```python
from build123d import *

# Parameters (mm, degrees)
SKETCH2_W               = 12.7
SKETCH2_H               = 6.35
BOSS_EXTRUDE1_DEPTH     = 9.525
EXTRUDE_THIN1_DEPTH     = 9.525
SKETCH4_R               = 4.370013209
CUT_EXTRUDE1_DEPTH      = 9.292796384
CUT_EXTRUDE1_DEPTH_BACK = 9.129454628
EXTRUDE_THIN3_DEPTH     = 1.27


with BuildPart() as part:
    # Sketch2 → Boss-Extrude1 (new body)
    with BuildSketch(Plane(origin=(0, 0, 0), x_dir=(1, 0, 0), z_dir=(0, 1, 0))):
        with Locations((0, -3.175)):
            Rectangle(SKETCH2_W, SKETCH2_H)
    extrude(amount=-BOSS_EXTRUDE1_DEPTH)

    # Sketch3 → Extrude-Thin1 (add)
    with BuildSketch(Plane(origin=(0, 0, 0), x_dir=(1, 0, 0), z_dir=(0, 1, 0))):
        with BuildLine():
            ThreePointArc((-6.979657819, -9.309768687), (0.081670878, -7.62), (7.142999576, -9.309768687))
            Line((7.142999576, -9.309768687), (8.292796384, -7.044913879))
            ThreePointArc((8.292796384, -7.044913879), (0.081670878, -5.08), (-8.129454628, -7.044913879))
            Line((-8.129454628, -7.044913879), (-6.979657819, -9.309768687))
        make_face()
    extrude(amount=-EXTRUDE_THIN1_DEPTH)

    # Sketch4 → Cut-Extrude1 (cut, two sides)
    with BuildSketch(Plane(origin=(0, 0, 0), x_dir=(0, 0, -1), z_dir=(1, 0, 0))) as cut_extrude1_sk:
        with Locations((-1.517033844, -4.7625)):
            Circle(SKETCH4_R)
    extrude(amount=CUT_EXTRUDE1_DEPTH, mode=Mode.SUBTRACT)
    extrude(cut_extrude1_sk.sketch, amount=-CUT_EXTRUDE1_DEPTH_BACK, mode=Mode.SUBTRACT)

    # Sketch6 → Extrude-Thin3 (add)
    with BuildSketch(Plane.XY):
        with BuildLine():
            ThreePointArc((-6.433087898, 0), (-0.041543949, 6.391543949), (6.35, 0))
            Line((6.35, 0), (5.08, 0))
            ThreePointArc((5.08, 0), (-0.041543949, 5.121543949), (-5.163087898, 0))
            Line((-5.163087898, 0), (-6.433087898, 0))
        make_face()
    extrude(amount=EXTRUDE_THIN3_DEPTH)


solid = part.part
```
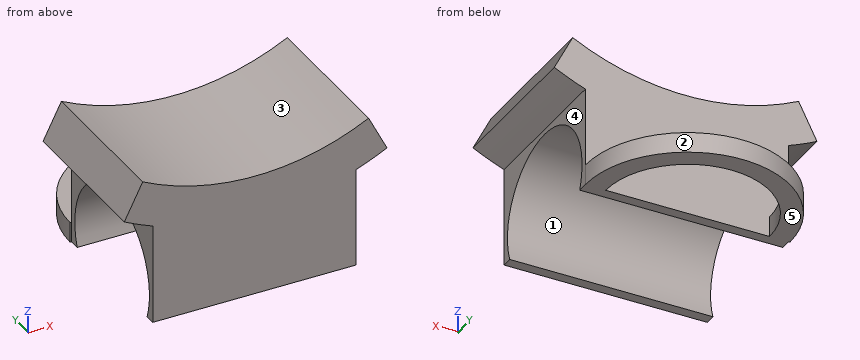
Verification items for the finished model (mm, model axes). Face numbers are marked on the shaded views. A direction names the side the tool comes from. Round coordinates to 2 decimals unless told otherwise and drop trailing zeros. Write each loop counter-clockwise with the first axis right and the second up, starting at its lowest first coordinate (ties: lowest second). Pieces come first, ordered by that corner, then holes. Notation, with made-up numbers: (67.5, -10) -> (125.5, -10) arc R20 cw to (125.5, 26) -> close; hole circle Ø2 at (57, -0.5). An arc over 180 degrees is marked (long way). Write each question's results on one line, items separated by ' | '. Start each with the question number.
1. Material ranges on probe 1 along Y at (x, z) = (-5, 1.5) (3 decimals); probe 2 along Z at (x, y) = (2.5, 5.5); probe 3 along X at (y, z) = (-7.75, 4.75), recorded low to high. Write a range as from..to.
2. Cross-section at B-B (y = 2.25). Enter the section's corners in (x, z), then the cut area to 3 significant figures.
3. Depth check by flat-ended pin: P1, Ø3, axis at x = -4, z = 5, coming from the +Y side; P2, Ø1.9, axis at y = -7, z = 2, coming from the +X side; P3, Ø5, axis at x = 4.5, y = -2.5, coming from the +Z side; P4, Ø2, axis at x = -1, y = -4, coming from the -Z side. Enter the tip coordinate at first touch or a pass-through.
4. Draft check along Z on the marked faces 1, 2 and 3. Enter one of: +Z half, -Z half, draft (parallel to the pull), parting line (faces both ways), or undercut.
5. Cross-section at C-C (z = 4.25). Enter the section's corners in (x, y) (3 decimals), then the cut area to 3 significant figures.
6. Cross-section at A-A (x = 2.5). Enter the section's corners in (y, z) (1 decimal).
7. Set-up check for the marked faces 4 and 5: record each of +Z, -Z, +X, -X, +Y, -Y from which the full face is reachable in a straight line by a thin tool's end or side.
8. Cross-section at D-D (y = -3.75). Enter the section's corners in (x, z).
Solutions:
1) probe 1: y = -9.525..-9.132, -0.393..0 | probe 2: z = 0..1.27 | probe 3: x = -6.35..6.35
2) outline: (-6.02, 0) -> (-4.64, 0) -> (-4.64, 1.27) -> (-6.02, 1.27) -> close; (4.56, 0) -> (5.94, 0) -> (5.94, 1.27) -> (4.56, 1.27) -> close | area: 3.51 mm2
3) P1: stops at y = 0 | P2: passes through | P3: stops at z = 9.24 | P4: stops at z = 5.52
4) face 1: undercut | face 2: draft | face 3: +Z half
5) outline: (-6.35, -9.525) -> (6.35, -9.525) -> (6.35, -8.172) -> (-6.35, -8.172) -> close; (-6.35, -1.353) -> (6.35, -1.353) -> (6.35, 0) -> (-6.35, 0) -> close | area: 34.4 mm2
6) outline: (-9.5, 0) -> (-8.9, 0) arc R4.4 cw (long way) to (-0.7, 0) -> (0, 0) -> (0, 7.8) -> (-9.5, 7.8) -> close; (4.4, 0) -> (5.9, 0) -> (5.9, 1.3) -> (4.4, 1.3) -> close
7) face 4: -Z, +X, +Y, -Y | face 5: -Z, +X, -X, +Y, -Y
8) outline: (-8.13, 7.04) arc R18.14 ccw to (-6.35, 6.26) -> (-6.35, 5.77) -> (6.35, 5.77) -> (6.35, 6.2) arc R18.14 ccw to (8.29, 7.04) -> (7.14, 9.31) arc R15.6 cw to (-6.98, 9.31) -> close
